```python
from build123d import *

# Parameters (mm, degrees)
F0_W     = 150
F0_H     = 2
F2_R     = 26
F3_DEPTH = 10
F4_R     = 24
F5_DEPTH = 13


with BuildPart() as f1:
    # F0 (on Right) → F1 (revolve)
    with BuildSketch(Plane.YZ):
        with Locations((0, -27)):
            Rectangle(F0_W, F0_H)
    revolve(axis=Axis((0, 25.8125, 0), (0, 1, 0)))

    # F2 (on face) → F3 (join, symmetric)
    with BuildSketch(Plane(origin=(0, 75, 0), x_dir=(-1, 0, 0), z_dir=(0, 1, 0))):
        Circle(F2_R)
    extrude(amount=F3_DEPTH, both=True)

    # F4 (on face) → F5 (cut)
    with BuildSketch(Plane(origin=(0, 85, 0), x_dir=(-1, 0, 0), z_dir=(0, 1, 0))):
        Circle(F4_R)
    extrude(amount=-F5_DEPTH, mode=Mode.SUBTRACT)


solid = f1.part
```
Work out the finished part from the listing and answer in its coordinate system (mm). A direction names the side the tool comes from. Give positions to 0.01 mm unless a question says otherwise; leave off trailing zeros. Order: outer loops, then holes, each group sorted by start corner. A loop starts at its lowest first (then second) coordinate and runs counter-clockwise, first axis right, second up. Notation, with made-up numbers: M -34.5,-22.5 L -27.5,-22.5 A22 ccw -27.5,9.5 Z; hole C 23.5,-3.75 d6. An arc over 180 degrees is marked long. Return JSON: item names as keys, results as strings.
1) Section C-C, the plane x = 0 is taken. Write down the section's boundary in (y, z).
Resolved:
{"outline": "M -75,-28 L 75,-28 L 75,-26 L 85,-26 L 85,-24 L 72,-24 L 72,24 L 85,24 L 85,26 L 75,26 L 75,28 L -75,28 L -75,26 L 65,26 L 65,-26 L -75,-26 Z"}
2) Each of these flat-tipped pins is pushed along its axis until it touches: pin 1 (8 mm diameter, centred on y = 51.5, z = 11, fed in from +X); pin 2 (10 mm diameter, centred on y = 55.5, z = 14, fed in from +X); pin 3 (8 mm diameter, centred on y = -3, z = -17, fed in from -X). Where does it stop, or does it pass through?
Resolved:
{"pin 1": "x = 27.11", "pin 2": "x = 26.51", "pin 3": "x = -24.8"}
3) For a pull along Z with two mould halves and no side action, classify faces 4 (the flat face through (-8, 85, -23)), 5 (the flat face through (0, 72, 0)), 6 (the cylindrical face through (10.724, 1.05, -25.865)), 7 (the flat face through (0, 65, 0)) as +Z half, -Z half, draft (parallel to the pull), parting line (faces both ways), or undercut.
Resolved:
{"face 4": "draft", "face 5": "undercut", "face 6": "parting line", "face 7": "undercut"}
4) Section A-A, the plane z = 0 is taken. Write down the section's boundary in (x, y), plus the area to 3 significant figures.
Resolved:
{"outline": "M -28,-75 L -26,-75 L -26,65 L 26,65 L 26,-75 L 28,-75 L 28,75 L 26,75 L 26,85 L 24,85 L 24,72 L -24,72 L -24,85 L -26,85 L -26,75 L -28,75 Z", "area": "1,020 mm^2"}
5) Section B-B, the plane y = -52.5 is taken. Write down the section's boundary in (x, z), plus the area to 3 significant figures.
Resolved:
{"outline": "C 0,0 d56; hole C 0,0 d52", "area": "339 mm^2"}
6) Straight lines are drawn through the part: line 1 along X through (y, z) = (-11, 0); line 2 along Z through (x, y) = (0, 77); line 3 along X through (y, z) = (59.5, -14). For each, find the intervals that lie inside material, in ascending order. Write a range as [from, to].
Resolved:
{"line 1": "[-28, -26], [26, 28]", "line 2": "[-26, -24], [24, 26]", "line 3": "[-24.25, -21.91], [21.91, 24.25]"}
7) A tool of negligible diameter and unlimited length cuts with its end or side. For faces 1 (the flat face through (8, 75, -25)), 2 (the flat face through (8, -75, -25)), 3 (the cylindrical face through (10, -4, -24)), from which of +Z, -Z, +X, -X, +Y, -Y can it reach the whole face along a straight path? Write none if from no direction.
Resolved:
{"face 1": "+Y", "face 2": "+Z, -Z, +X, -X, -Y", "face 3": "-Y"}
